Build history of the part. All positions in model axes, mm. A direction names the side the tool comes from. Give positions to 0.01 mm unless a question says otherwise; leave off trailing zeros. Order: outer loops, then holes, each group sorted by start corner. A loop starts at its lowest first (then second) coordinate and runs counter-clockwise, first axis right, second up. Notation, with made-up numbers: (85.25, 65.5) - (96.25, 65.5) arc R34 ccw to (96.25, 100.5) - close; hole circle Ø7 at (17.5, 40). An arc over 180 degrees is marked (long way). Use a Markdown table: item, result. Add a question column.
(1) Slice it at A-A (y = 2.75). Write the cut outline in (x, z), then the cut area to 3 significant figures.
(2) Wall check: line 1 (X direction, y = 8.25, z = -6.75); line 2 (Z direction, x = 7.5, y = 14); line 3 (Y direction, x = 41, z = -3.5). Give the ranges that are in metal, low to high.
(3) Slice it at B-B (z = -6.5). Write the cut outline in (x, y).
(4) Slice it at C-C (x = 60). Write the cut outline in (y, z), then the cut area to 3 significant figures.
(5) Flat gauge pins, fed straight in: pin 1 (1.5 mm diameter, centred on y = 4, z = -11, fed in from -X); pin 2 (6 mm diameter, centred on y = 7, z = -2.5, fed in from +X); pin 3 (3 mm diameter, centred on y = 5.5, z = -12, fed in from -X); pin 4 (2.5 mm diameter, centred on x = 0, z = -6.5, fed in from -Y). Where does each tip first touch, or does it go through?
(6) Which spindle directions (+Z, -Z, +X, -X, +Y, -Y) get a long thin tool onto all of the face, cutting with end or side? Do faces 5 (the face through (34, 16.5, -7)), 6 (the face through (14.5, 7, -11)), 7 (the face through (6.5, 7, -6)). Say none if no direction does.
(7) Slice it at D-D (z = -2.25). Write the cut outline in (x, y), then the cut area to 3 significant figures.
(8) Mould opens along Z. For faces 1 (the face through (54.5, 7, -11)), 2 (the face through (34, 15, 0)), 3 (the face through (10, 7, -9)), 4 (the face through (59, 7, -4)) say: +Z half, -Z half, draft (parallel to the pull), parting line (faces both ways), or undercut.
from build123d import *

# Parameters (mm, degrees)
BOSS_EXTRU_1_DEPTH      = 16.5
ESQUISSE2_R             = 2
ENL_V_MAT_EXTRU_1_DEPTH = 22
ENL_V_MAT_EXTRU_2_DEPTH = 14.5


with BuildPart() as part:
    # Esquisse1 → Boss.-Extru.1 (new body)
    with BuildSketch(Plane(origin=(0, 0, 0), x_dir=(1, 0, 0), z_dir=(0, 1, 0))):
        with BuildLine():
            Line((0, 0), (69, 0))
            ThreePointArc((69, 0), (75.5, 6.5), (69, 13))
            Line((69, 13), (0, 13))
            ThreePointArc((0, 13), (-6.5, 6.5), (0, 0))
        make_face()
    extrude(amount=BOSS_EXTRU_1_DEPTH)

    # Esquisse2 → Enlèv. mat.-Extru.1 (cut)
    with BuildSketch(Plane(origin=(0, 16.5, 0), x_dir=(1, 0, 0), z_dir=(0, 1, 0))):
        with Locations(Location((0, 6.5, 0), (0, 0, 270))):
            Circle(ESQUISSE2_R)
        with Locations(Location((69, 6.5, 0), (0, 0, 270))):
            Circle(ESQUISSE2_R)
    extrude(amount=-ENL_V_MAT_EXTRU_1_DEPTH, mode=Mode.SUBTRACT)

    # Esquisse3 → Enlèv. mat.-Extru.2 (cut)
    with BuildSketch(Plane(origin=(0, 0, 0), x_dir=(-1, 0, 0), z_dir=(0, -1, 0))):
        Polygon((-54.5, 13), (-54.5, 9), (-62.5, 9), (-62.5, 4), (-54.5, 4), (-54.5, 0), (-14.5, 0), (-14.5, 4), (-6.5, 4), (-6.5, 9), (-14.5, 9), (-14.5, 13), align=None)
    extrude(amount=-ENL_V_MAT_EXTRU_2_DEPTH, mode=Mode.SUBTRACT)


solid = part.part
Solution:
| question | item | result |
|---|---|---|
| 1 | outline | (0, -13) - (14.5, -13) - (14.5, -9) - (6.5, -9) - (6.5, -4) - (14.5, -4) - (14.5, 0) - (0, 0) arc R6.5 ccw to start; (54.5, -13) - (69, -13) arc R6.5 ccw to (69, 0) - (54.5, 0) - (54.5, -4) - (62.5, -4) - (62.5, -9) - (54.5, -9) - close; hole circle Ø4 at (0, -6.5); hole circle Ø4 at (69, -6.5) |
| 1 | area | 405 mm2 |
| 2 | line 1 | -6.5 to -1.98, 1.98 to 6.5, 62.5 to 67.02, 70.98 to 75.5 |
| 2 | line 2 | -13 to -9, -4 to 0 |
| 2 | line 3 | 14.5 to 16.5 |
| 3 | outline | (-6.5, 0) - (-2, 0) - (-2, 16.5) - (-6.5, 16.5) - close; (2, 0) - (6.5, 0) - (6.5, 14.5) - (62.5, 14.5) - (62.5, 0) - (67, 0) - (67, 16.5) - (2, 16.5) - close; (71, 0) - (75.5, 0) - (75.5, 16.5) - (71, 16.5) - close |
| 4 | outline | (0, -13) - (16.5, -13) - (16.5, 0) - (0, 0) - (0, -4) - (14.5, -4) - (14.5, -9) - (0, -9) - close |
| 4 | area | 142 mm2 |
| 5 | pin 1 | x = -5.31 |
| 5 | pin 2 | x = 75.42 |
| 5 | pin 3 | x = -5.12 |
| 5 | pin 4 | through |
| 6 | face 5 | +Z, -Z, +X, -X, +Y |
| 6 | face 6 | +Z, -Z, -Y |
| 6 | face 7 | -Y |
| 7 | outline | (-4.92, 0) - (14.5, 0) - (14.5, 14.5) - (54.5, 14.5) - (54.5, 0) - (73.92, 0) - (73.92, 16.5) - (-4.92, 16.5) - close |
| 7 | area | 721 mm2 |
| 8 | face 1 | draft |
| 8 | face 2 | +Z half |
| 8 | face 3 | undercut |
| 8 | face 4 | undercut |
